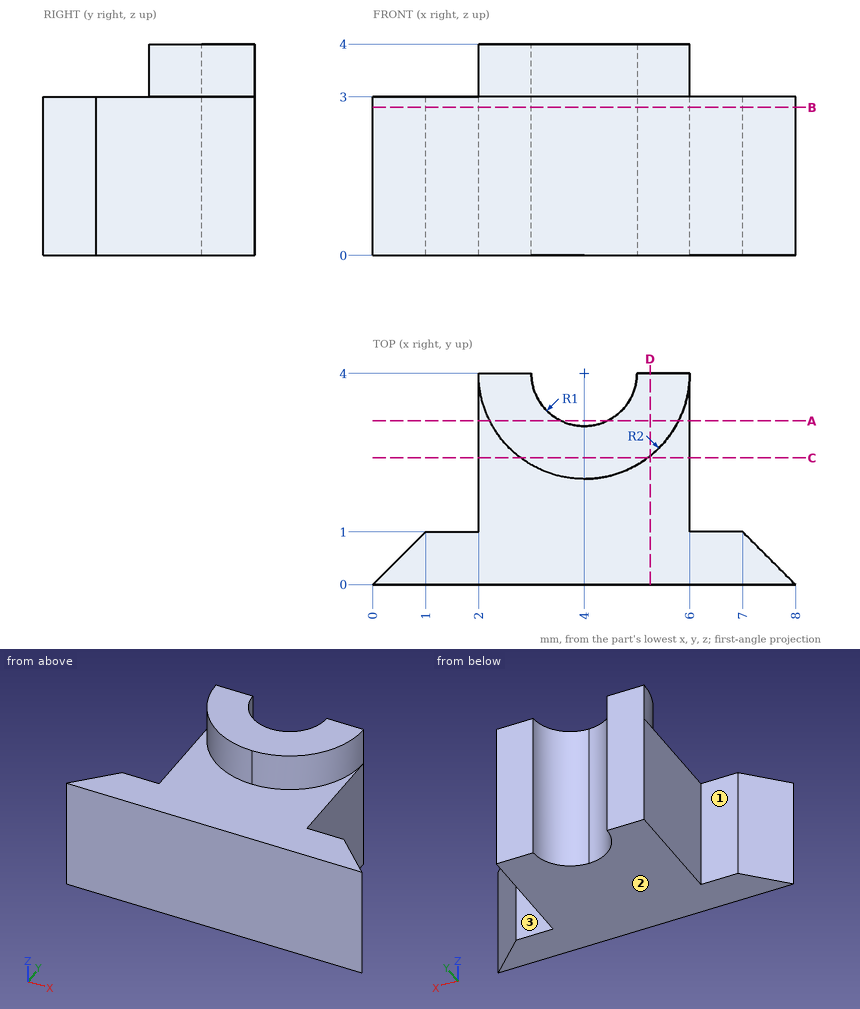
Drawing for the job (mm, zero at the part's lowest x, y, z). A direction names the side the tool comes from. Coordinates: 2 decimals unless noted, no trailing zeros. Order: outer loops, then holes, each group sorted by start corner. A loop starts at its lowest first (then second) coordinate and runs counter-clockwise, first axis right, second up. Notation, with made-up numbers: (21.25, 71) -> (65.25, 71) arc R5 cw to (65.25, 76) -> close; hole circle Ø9 at (66.25, 52). An arc over 180 degrees is marked (long way). Return JSON: item names as keys, results as strings.
Item 1: Slice it at B-B (z = 2.8). Write the cut outline in (x, y).
Model answer:
{"outline": "(0, 0) -> (8, 0) -> (7, 1) -> (6, 1) -> (6, 4) -> (5, 4) arc R1 cw to (3, 4) -> (2, 4) -> (2, 1) -> (1, 1) -> close"}
Item 2: Slice it at A-A (y = 3.1). Write the cut outline in (x, z).
Model answer:
{"outline": "(2, 0) -> (3.56, 0) -> (3.56, 4) -> (2.21, 4) -> (2.21, 3) -> (2, 3) -> close; (4.44, 0) -> (6, 0) -> (6, 3) -> (5.79, 3) -> (5.79, 4) -> (4.44, 4) -> close"}
Item 3: 3-axis set-ups, long thin cutter, end or side, ignore diameter. For the marked faces 1, 2 and 3: which of +Z, -Z, +X, -X, +Y, -Y reach the whole face in a straight line?
Model answer:
{"face 1": "+Z, -Z, -X, +Y", "face 2": "-Z, +X, -X, +Y, -Y", "face 3": "+Z, -Z, +X, +Y"}
Item 4: Wall check: line 1 along Z through (x, y) = (3.25, 1.6); line 2 along X through (y, z) = (2.4, 1.2); line 3 along X through (y, z) = (3.6, 2.2). Give the ranges that are in metal, low to high. Write a range as from..to.
Model answer:
{"line 1": "z = 0..3", "line 2": "x = 2..6", "line 3": "x = 2..3.08, 4.92..6"}
Item 5: Pin check, flat tips, straight feed: P1, Ø2, axis at x = 6, y = 1, coming from the +Z side; P2, Ø0.9, axis at y = 2, z = 1, coming from the +X side; P3, Ø0.8, axis at x = 1.5, z = 2, coming from the +Y side. Stop position of each tip, or through.
Model answer:
{"P1": "stops at z = 3", "P2": "stops at x = 6", "P3": "stops at y = 1"}
Item 6: Slice it at D-D (x = 5.25). Write the cut outline in (y, z).
Model answer:
{"outline": "(0, 0) -> (4, 0) -> (4, 4) -> (2.44, 4) -> (2.44, 3) -> (0, 3) -> close"}
Item 7: Slice it at C-C (y = 2.4). Write the cut outline in (x, z), then the cut area to 3 significant figures.
Model answer:
{"outline": "(2, 0) -> (6, 0) -> (6, 3) -> (5.2, 3) -> (5.2, 4) -> (2.8, 4) -> (2.8, 3) -> (2, 3) -> close", "area": "14.4 mm²"}
